Verification items for the finished model (mm, model axes). A direction names the side the tool comes from. Give positions to 0.01 mm unless a question says otherwise; leave off trailing zeros. Loops run counter-clockwise (first coordinate to the right, second up) from the corner with the lowest first, then second, coordinate; pieces in that order, holes last. Notation, with made-up numbers: M 64.5,83.5 L 117.5,83.5 A21 ccw 117.5,89.5 Z; hole C -28.5,-8.5 d6. An arc over 180 degrees is marked long. Write each question's results on one line, items separated by ' | '. Start each with the question number.
```python
from build123d import *

# Parameters (mm, degrees)
F0_W     = 20
F0_H     = 20
F1_DEPTH = 700
F2_R     = 2
F3_T     = 2
F4_R     = 2
F5_R     = 2.5
F6_DEPTH = 25.2


# Not quite as in the source:
# - a shell that OpenCascade refuses in one call is made with other operations: the cavity is built on its own and cut out


with BuildPart() as f1:
    # F0 (on Top) → F1 (new body)
    with BuildSketch(Plane.XY):
        Rectangle(F0_W, F0_H)
    extrude(amount=F1_DEPTH)

    # F2
    f2_edges = [f1.edges().sort_by_distance(p)[0] for p in [
        (-10, 10, 350),
        (-10, -10, 350),
        (10, -10, 350),
        (10, 10, 350),
    ]]
    fillet(f2_edges, radius=F2_R)

    # F3: shell of thickness 2, made by hand


with BuildPart() as f3_core1:
    # F3_t2: copy of F1
    add(f1.part)

    # the walls: a layer under each face that stays
    f3_faces = [f3_core1.faces().sort_by_distance(p)[0] for p in [
        (0, -10, 350),
        (-10, 0, 350),
        (10, 0, 350),
        (0, 10, 350),
    ]]
    thicken(f3_faces, amount=-F3_T, mode=Mode.SUBTRACT)


with BuildPart() as f1_1:
    add(f1.part)

    # what is left inside the walls is the cavity
    f3_cavity = [f3_core1.part.solids().sort_by_distance(p)[0] for p in [
        (-7.98, 0, 466.666667),
    ]]
    add(f3_cavity, mode=Mode.SUBTRACT)

    # F4
    f4_edges = [f1_1.edges().sort_by_distance(p)[0] for p in [
        (-8, 8, 350),
        (-8, -8, 350),
        (8, -8, 350),
        (8, 8, 350),
    ]]
    fillet(f4_edges, radius=F4_R)

    # F5 (on face) → F6 (cut)
    with BuildSketch(Plane(origin=(0, 10, 0), x_dir=(-1, 0, 0), z_dir=(0, 1, 0))):
        with Locations((0, 10)):
            Circle(F5_R)
    extrude(amount=-F6_DEPTH, mode=Mode.SUBTRACT)


solid = f1_1.part
```
1. Section check B-B, the plane z = 143. Record the boundary of the cut face in (x, y).
2. Set-up check for faces 1 (the face through (0, -8, 345)), 2 (the face through (0, -10, 345)): record each of +Z, -Z, +X, -X, +Y, -Y from which the full face is reachable in a straight line by a thin tool's end or side.
3. Release check for a two-part mould opening along X. For faces 3 (the face through (-9, 0, 0)), 4 (the face through (-10, 0, 345)), 5 (the face through (0, 8, 345)) record: released by +X, released by -X, zero draft, split by the parting line, or undercut.
4. Thickness scan on probe 1 along Y at (x, z) = (4, 257); probe 2 along Z at (x, y) = (0, 9.3). Record the ranges inside material, lowest first.
5. Depth check by flat-ended pin: pin 1 Ø6 at (x, y) = (1.5, -3) entering from +Z. Enter the tip coordinate at first touch or a pass-through.
6. Section check A-A, the plane y = 3. Record the boundary of the cut face in (x, z), plus the area to 3 significant figures.
Filled sheet:
1) outline: M -10,-8 A2 ccw -8,-10 L 8,-10 A2 ccw 10,-8 L 10,8 A2 ccw 8,10 L -8,10 A2 ccw -10,8 Z; hole M -8,-6 A2 ccw -6,-8 L 6,-8 A2 ccw 8,-6 L 8,6 A2 ccw 6,8 L -6,8 A2 ccw -8,6 Z
2) face 1: +Z, -Z | face 2: +Z, -Z, +X, -X, -Y
3) face 3: zero draft | face 4: released by -X | face 5: undercut
4) probe 1: -10 to -8, 8 to 10 | probe 2: 0 to 7.5, 12.5 to 700
5) pin 1: through
6) outline: M -10,0 L -8,0 L -8,700 L -10,700 Z; M 8,0 L 10,0 L 10,700 L 8,700 Z | area: 2,800 mm2
